Here's how the part is built. I have some questions about the finished solid (model axes, mm). Coordinates: 2 decimals unless noted, no trailing zeros. Write each loop counter-clockwise with the first axis right and the second up, starting at its lowest first coordinate (ties: lowest second). Pieces come first, ordered by that corner, then holes. Notation, with made-up numbers: M 1,53 L 13,53 A12 cw 13,71 Z; hole C 24.5,-5.75 d4. An arc over 180 degrees is marked long. Use one line per item in the form item = value. Start each with the question number.
1. I want a section at A-A, the plane x = -150. List the corners of the cut face in (y, z) for me.
2. Please list where these lines run through material, in increasing order: line 1 along X through (y, z) = (-0.8, 27); line 2 along Z through (x, y) = (-150, -0.95); line 3 along X through (y, z) = (-0.5, 20). Write a range as [from, to].
3. I want a section at B-B, the plane y = -0.8. List the corners of the cut face in (x, z) for me, plus the area to 3 significant figures.
4. Thinking about a two-plate mould opening in X: for faces 1 (the face through (-3, -2.5, 1)), 2 (the face through (-146.185, -1.232, 31.201)), which applies, released by +X, released by -X, zero draft, split by the parting line, or undercut?
from build123d import *

# Parameters (mm, degrees)
F0_W     = 390
F0_H     = 120
F0_W_2   = 50
F0_H_2   = 20
F0_R     = 4
F1_DEPTH = 2.5


with BuildPart() as f1:
    # F0 (on Front) → F1 (new body)
    with BuildSketch(Plane.XZ):
        Rectangle(F0_W, F0_H)
        with Locations((-20, -10)):
            Rectangle(F0_W_2, F0_H_2, mode=Mode.SUBTRACT)
        with Locations((-20, 20)):
            Rectangle(F0_W_2, F0_H_2, mode=Mode.SUBTRACT)
        with Locations((-150, 30)):
            Circle(F0_R, mode=Mode.SUBTRACT)
    extrude(amount=F1_DEPTH)


solid = f1.part
Answer list:
q1.outline = M -2.5,-60 L 0,-60 L 0,26 L -2.5,26 Z; M -2.5,34 L 0,34 L 0,60 L -2.5,60 Z
q2.line_1 = [-195, -152.65], [-147.35, -45], [5, 195]
q2.line_2 = [-60, 26], [34, 60]
q2.line_3 = [-195, -45], [5, 195]
q3.outline = M -195,-60 L 195,-60 L 195,60 L -195,60 Z; hole C -150,30 d8; hole M -45,-20 L 5,-20 L 5,0 L -45,0 Z; hole M -45,10 L 5,10 L 5,30 L -45,30 Z
q3.area = 44,700 mm²
q4.face_1 = zero draft
q4.face_2 = undercut
